from build123d import *

# Parameters (mm, degrees)
SALIENTE_EXTRUIR1_DEPTH = 6
SALIENTE_EXTRUIR2_DEPTH = 2
CROQUIS3_W              = 12
CROQUIS3_H              = 4.5
SALIENTE_EXTRUIR3_DEPTH = 3.5
CROQUIS4_W              = 17
CROQUIS4_H              = 12
SALIENTE_EXTRUIR4_DEPTH = 9.5
CROQUIS5_W              = 19
CROQUIS5_H              = 13
CROQUIS6_W              = 10.5
CROQUIS6_H              = 9
REDONDEO1_R             = 0.5
CORTAR_EXTRUIR1_DEPTH   = 3
SALIENTE_EXTRUIR5_DEPTH = 3


with BuildPart() as part:
    # Croquis1 → Saliente-Extruir1 (new body)
    with BuildSketch(Plane.XY):
        with BuildLine():
            Line((-4, 3.5), (4, 3.5))
            ThreePointArc((4, 3.5), (7.5, 0), (4, -3.5))
            Line((4, -3.5), (-4, -3.5))
            ThreePointArc((-4, -3.5), (-7.5, 0), (-4, 3.5))
        make_face()
    extrude(amount=SALIENTE_EXTRUIR1_DEPTH)

    # Croquis2 → Saliente-Extruir2 (add)
    with BuildSketch(Plane.XY.offset(6)):
        with BuildLine():
            Line((-4, 3.5), (4.25, 3.5))
            ThreePointArc((4.25, 3.5), (7.75, 0), (4.25, -3.5))
            Line((4.25, -3.5), (-4, -3.5))
            ThreePointArc((-4, -3.5), (-7.5, 0), (-4, 3.5))
        make_face()
    extrude(amount=SALIENTE_EXTRUIR2_DEPTH)

    # Croquis3 → Saliente-Extruir3 (add)
    with BuildSketch(Plane(origin=(0, 0, 0), x_dir=(-1, 0, 0), z_dir=(0, 0, -1))):
        Rectangle(CROQUIS3_W, CROQUIS3_H)
    extrude(amount=SALIENTE_EXTRUIR3_DEPTH)

    # Croquis4 → Saliente-Extruir4 (add)
    with BuildSketch(Plane(origin=(0, 0, -3.5), x_dir=(-1, 0, 0), z_dir=(0, 0, -1))):
        Rectangle(CROQUIS4_W, CROQUIS4_H)
    extrude(amount=SALIENTE_EXTRUIR4_DEPTH)

    # Croquis5 → Recubrir1 section 0
    with BuildSketch(Plane(origin=(0, 0, -13), x_dir=(-1, 0, 0), z_dir=(0, 0, -1))):
        Rectangle(CROQUIS5_W, CROQUIS5_H)
    # Croquis6 → Recubrir1 section 1
    with BuildSketch(Plane(origin=(0, 0, -36.5), x_dir=(-1, 0, 0), z_dir=(0, 0, -1))):
        Rectangle(CROQUIS6_W, CROQUIS6_H)
    loft()

    # Redondeo1
    redondeo1_edges = [part.edges().sort_by_distance(p)[0] for p in [
        (-8.5, 0, -3.5),
        (-8.5, -6, -8.25),
        (0, 6, -3.5),
        (-8.5, 6, -8.25),
        (8.5, 0, -3.5),
        (8.5, 6, -8.25),
        (0, -6, -3.5),
        (8.5, -6, -8.25),
    ]]
    fillet(redondeo1_edges, radius=REDONDEO1_R)

    # Croquis7 → Cortar-Extruir1 (cut)
    with BuildSketch(Plane.XY.offset(8)):
        with BuildLine():
            Line((-3, 1.25), (3, 1.25))
            ThreePointArc((3, 1.25), (4.25, 0), (3, -1.25))
            Line((3, -1.25), (-3, -1.25))
            ThreePointArc((-3, -1.25), (-4.25, 0), (-3, 1.25))
        make_face()
    extrude(amount=-CORTAR_EXTRUIR1_DEPTH, mode=Mode.SUBTRACT)

    # Croquis8 → Saliente-Extruir5 (add)
    with BuildSketch(Plane.XY.offset(5)):
        with BuildLine():
            Line((-2.665643122, 0.419863202), (2.704700164, 0.419863202))
            ThreePointArc((2.704700164, 0.419863202), (3.124563366, 0), (2.704700164, -0.419863202))
            Line((2.704700164, -0.419863202), (-2.665643122, -0.419863202))
            ThreePointArc((-2.665643122, -0.419863202), (-3.085506324, 0), (-2.665643122, 0.419863202))
        make_face()
    extrude(amount=SALIENTE_EXTRUIR5_DEPTH)


solid = part.part
Can you work these out from the model? Positions are in its coordinate system, mm. A direction names the side the tool comes from. Give positions to 0.01 mm unless a question says otherwise; leave off trailing zeros. Order: outer loops, then holes, each group sorted by start corner. A loop starts at its lowest first (then second) coordinate and runs counter-clockwise, first axis right, second up. Notation, with made-up numbers: M 82,20 L 107,20 A16 cw 107,30 Z; hole C 88,33.5 d5. An arc over 180 degrees is marked long. Use a Markdown table: item, result. Add a question column.
Item 1: Suppose I cut it at A-A (z = -10.5). List the corners of the cut face in (x, y) for me.
Item 2: Will these pins go through, and if not, where does the flat tip stop? pin 1 (3 mm diameter, centred on x = -6, z = -30.5, fed in from +Y); pin 2 (3.5 mm diameter, centred on x = 0.5, z = 6.5, fed in from +Y); pin 3 (2 mm diameter, centred on x = 7.5, z = -8, fed in from -Y); pin 4 (1.5 mm diameter, centred on x = -7, z = -1.5, fed in from -Y).
Item 3: We'd pull the mould along Z, two halves only. Please class faces 5 (the cylindrical face through (-4.25, -0.03, 6.52)), 6 (the flat face through (0, 0, 8)), 7 (the flat face through (0, 2.25, -2)): +Z half, -Z half, draft (parallel to the pull), parting line (faces both ways), or undercut.
Item 4: If I drill on L1, parallel to X at y = 1, z = -10.5; L2, parallel to Y at x = -1, z = 4.5; L3, parallel to Y at x = -0.25, z = -12, over which ranges is the centre line in solid material (lowest first)? Write a range as [from, to].
Item 5: Suppose I cut it at B-B (z = 3). List the corners of the cut face in (x, y) for me.
Item 6: For faces 1 (the cylindrical face through (-7.5, -0.1, 3.9)), 2 (the flat face through (0, 6, -8)), 3 (the flat face through (0, -3.5, 4)), 4 (the flat face through (0, 0.42, 6)), which set-ups out of +Z, -Z, +X, -X, +Y, -Y let a thin tool reach every point of the face, with its end or its side?
Answer sheet:
| question | item | result |
|---|---|---|
| 1 | outline | M -8.5,-5.5 A0.5 ccw -8,-6 L 8,-6 A0.5 ccw 8.5,-5.5 L 8.5,5.5 A0.5 ccw 8,6 L -8,6 A0.5 ccw -8.5,5.5 Z |
| 2 | pin 1 | stops at y = 5.14 |
| 2 | pin 2 | stops at y = 3.5 |
| 2 | pin 3 | stops at y = -6 |
| 2 | pin 4 | passes through |
| 3 | face 5 | draft |
| 3 | face 6 | +Z half |
| 3 | face 7 | undercut |
| 4 | L1 | x = [-8.5, 8.5] |
| 4 | L2 | y = [-3.5, 3.5] |
| 4 | L3 | y = [-6, 6] |
| 5 | outline | M -4,-3.5 L 4,-3.5 A3.5 ccw 4,3.5 L -4,3.5 A3.5 ccw Z |
| 6 | face 1 | +Z, -X |
| 6 | face 2 | +Z, +X, -X, +Y |
| 6 | face 3 | +Z, +X, -X, -Y |
| 6 | face 4 | +Z |
